from build123d import *

# Parameters (mm, degrees)
SKETCH1_W                          = 155
SKETCH1_H                          = 209.16
BACKPLATE_DEPTH                    = 1.016
IO_SHIELD_CUTOUT_REACH             = 262.334
SKETCH2_W                          = 44.45
SKETCH2_H                          = 158.75
FILLET1_R                          = 0.99
EXPANSION_CARD_CUTOUT_REACH        = 262.334
SKETCH5_W                          = 15
SKETCH5_H                          = 104
SKETCH5_W_2                        = 60.69
SKETCH5_H_2                        = 16
CONVERT_SOLID2_START               = -0.1524
CONVERT_SOLID2_OUTLINE_W           = 155
CONVERT_SOLID2_OUTLINE_H           = 209.16
CONVERT_SOLID2_OUTLINE_W_2         = 15
CONVERT_SOLID2_OUTLINE_H_2         = 104
CONVERT_SOLID2_OUTLINE_W_3         = 60.69
CONVERT_SOLID2_OUTLINE_H_3         = 16
CONVERT_SOLID2_DEPTH               = 0.1524
FILLET2_R                          = 3.048
EXPANSION_CARD_TABS_REACH          = 262.335
SKETCH33_W                         = 15
SKETCH33_H                         = 2
LPATTERN1_COUNT                    = 3
LPATTERN1_PITCH                    = 20.23
M3_CLEARANCE_HOLE_FRAME_MOUNTING_D = 3.4
PANEL_MOUNT_CABLE_CUTOUT_REACH     = 262.335
SKETCH42_W                         = 30.5
SKETCH42_H                         = 22
FILLET3_R                          = 1.5
TAP_DRILL_FOR_M3X0_5_TAP1_D        = 2.5
FILLET4_R                          = 2
FILLET5_R                          = 1
SPINE_MOUNTING_HOLES_D             = 3.2
SPINE_MOUNTING_HOLES_DEPTH         = 5
SPINE_MOUNTING_HOLES_TIP           = 0.96137699


# Read off the part's stored shape, not the designer's step: Convert-Solid2
with BuildPart() as part:
    # Sketch1 → backplate (new body)
    with BuildSketch(Plane.XY):
        with Locations((77.5, 104.58)):
            Rectangle(SKETCH1_W, SKETCH1_H)
    extrude(amount=BACKPLATE_DEPTH)

    # Sketch2 → io_shield_cutout (cut, up to next)
    with BuildSketch(Plane.XY.offset(1.016), mode=Mode.PRIVATE) as io_shield_cutout_sk1:
        with Locations((58.945, 81.955)):
            Rectangle(SKETCH2_W, SKETCH2_H)
    io_shield_cutout_tool1 = extrude(io_shield_cutout_sk1.sketch, amount=-IO_SHIELD_CUTOUT_REACH, mode=Mode.PRIVATE) & part.part
    add(io_shield_cutout_tool1.solids().sort_by_distance((58.945, 81.955, 1.016))[0], mode=Mode.SUBTRACT)

    # Fillet1
    fillet1_edges = [part.edges().sort_by_distance(p)[0] for p in [
        (36.72, 2.58, 0.508),
        (36.72, 161.33, 0.508),
        (81.17, 161.33, 0.508),
        (81.17, 2.58, 0.508),
    ]]
    fillet(fillet1_edges, radius=FILLET1_R)

    # Sketch5 → expansion-card-cutout (cut, up to next)
    with BuildSketch(Plane.XY.offset(1.016), mode=Mode.PRIVATE) as expansion_card_cutout_sk1:
        with Locations((103.88, 89)):
            Rectangle(SKETCH5_W, SKETCH5_H)
    expansion_card_cutout_tool1 = extrude(expansion_card_cutout_sk1.sketch, amount=-EXPANSION_CARD_CUTOUT_REACH, mode=Mode.PRIVATE) & part.part
    # Sketch5 → expansion-card-cutout (cut, up to next)
    with BuildSketch(Plane.XY.offset(1.016), mode=Mode.PRIVATE) as expansion_card_cutout_sk2:
        with Locations((121.835, 153)):
            Rectangle(SKETCH5_W_2, SKETCH5_H_2)
    expansion_card_cutout_tool2 = extrude(expansion_card_cutout_sk2.sketch, amount=-EXPANSION_CARD_CUTOUT_REACH, mode=Mode.PRIVATE) & part.part
    # Sketch5 → expansion-card-cutout (cut, up to next)
    with BuildSketch(Plane.XY.offset(1.016), mode=Mode.PRIVATE) as expansion_card_cutout_sk3:
        with Locations((124.2, 89)):
            Rectangle(SKETCH5_W, SKETCH5_H)
    expansion_card_cutout_tool3 = extrude(expansion_card_cutout_sk3.sketch, amount=-EXPANSION_CARD_CUTOUT_REACH, mode=Mode.PRIVATE) & part.part
    # Sketch5 → expansion-card-cutout (cut, up to next)
    with BuildSketch(Plane.XY.offset(1.016), mode=Mode.PRIVATE) as expansion_card_cutout_sk4:
        with Locations((144.52, 89)):
            Rectangle(SKETCH5_W, SKETCH5_H)
    expansion_card_cutout_tool4 = extrude(expansion_card_cutout_sk4.sketch, amount=-EXPANSION_CARD_CUTOUT_REACH, mode=Mode.PRIVATE) & part.part
    add(expansion_card_cutout_tool1.solids().sort_by_distance((103.88, 89, 1.016))[0], mode=Mode.SUBTRACT)
    add(expansion_card_cutout_tool2.solids().sort_by_distance((121.835, 153, 1.016))[0], mode=Mode.SUBTRACT)
    add(expansion_card_cutout_tool3.solids().sort_by_distance((124.2, 89, 1.016))[0], mode=Mode.SUBTRACT)
    add(expansion_card_cutout_tool4.solids().sort_by_distance((144.52, 89, 1.016))[0], mode=Mode.SUBTRACT)

    # Convert-Solid2 outline → Convert-Solid2 (add)
    with BuildSketch(Plane.XY.offset(CONVERT_SOLID2_START)):
        with Locations((77.5, 104.58)):
            Rectangle(CONVERT_SOLID2_OUTLINE_W, CONVERT_SOLID2_OUTLINE_H)
        with BuildLine():
            ThreePointArc((37.71, 2.58), (37.009964287, 2.869964287), (36.72, 3.57))
            Line((36.72, 3.57), (36.72, 160.34))
            ThreePointArc((36.72, 160.34), (37.009964287, 161.040035713), (37.71, 161.33))
            Line((37.71, 161.33), (80.18, 161.33))
            ThreePointArc((80.18, 161.33), (80.880035713, 161.040035713), (81.17, 160.34))
            Line((81.17, 160.34), (81.17, 3.57))
            ThreePointArc((81.17, 3.57), (80.880035713, 2.869964287), (80.18, 2.58))
            Line((80.18, 2.58), (37.71, 2.58))
        make_face(mode=Mode.SUBTRACT)
        with Locations((103.88, 89)):
            Rectangle(CONVERT_SOLID2_OUTLINE_W_2, CONVERT_SOLID2_OUTLINE_H_2, mode=Mode.SUBTRACT)
        with Locations((124.2, 89)):
            Rectangle(CONVERT_SOLID2_OUTLINE_W_2, CONVERT_SOLID2_OUTLINE_H_2, mode=Mode.SUBTRACT)
        with Locations((144.52, 89)):
            Rectangle(CONVERT_SOLID2_OUTLINE_W_2, CONVERT_SOLID2_OUTLINE_H_2, mode=Mode.SUBTRACT)
        with Locations((121.835, 153)):
            Rectangle(CONVERT_SOLID2_OUTLINE_W_3, CONVERT_SOLID2_OUTLINE_H_3, mode=Mode.SUBTRACT)
    extrude(amount=CONVERT_SOLID2_DEPTH)

    # Fillet2
    fillet2_edges = [part.edges().sort_by_distance(p)[0] for p in [
        (0, 0, 0.4318),
        (0, 209.16, 0.4318),
        (155, 209.16, 0.4318),
        (155, 0, 0.4318),
    ]]
    fillet(fillet2_edges, radius=FILLET2_R)

    # Sketch33 → expansion-card-tabs (cut, up to next)
    with BuildSketch(Plane.XY.offset(1.016), mode=Mode.PRIVATE) as expansion_card_tabs_sk1:
        with Locations((103.88, 32)):
            Rectangle(SKETCH33_W, SKETCH33_H)
    expansion_card_tabs_tool1 = extrude(expansion_card_tabs_sk1.sketch, amount=-EXPANSION_CARD_TABS_REACH, mode=Mode.PRIVATE) & part.part
    # Sketch33 → expansion-card-tabs (cut, up to next)
    with BuildSketch(Plane.XY.offset(1.016), mode=Mode.PRIVATE) as expansion_card_tabs_sk2:
        with Locations((103.88, 28.5)):
            Rectangle(SKETCH33_W, SKETCH33_H)
    expansion_card_tabs_tool2 = extrude(expansion_card_tabs_sk2.sketch, amount=-EXPANSION_CARD_TABS_REACH, mode=Mode.PRIVATE) & part.part
    expansion_card_tabs_1 = expansion_card_tabs_tool1.solids().sort_by_distance((103.88, 32, 1.016))[0]
    add(expansion_card_tabs_1, mode=Mode.SUBTRACT)
    expansion_card_tabs_2 = expansion_card_tabs_tool2.solids().sort_by_distance((103.88, 28.5, 1.016))[0]
    add(expansion_card_tabs_2, mode=Mode.SUBTRACT)
    expansion_card_tabs = expansion_card_tabs_1 + expansion_card_tabs_2  # expansion-card-tabs as one shape, for the pattern or mirror that repeats it

    # LPattern1: expansion-card-tabs ×3
    with Locations(*[(i * LPATTERN1_PITCH, 0, 0) for i in range(1, LPATTERN1_COUNT)]):
        add(expansion_card_tabs, mode=Mode.SUBTRACT)

    # M3 Clearance Hole frame mounting (through all)
    with Locations(Plane(origin=(0, 0, -0.1524), x_dir=(-1, 0, 0), z_dir=(0, 0, -1))):
        with Locations((-12.6, 7.025), (-141, 176.135), (-141, 7.025), (-12.6, 176.135)):
            Hole(M3_CLEARANCE_HOLE_FRAME_MOUNTING_D / 2)

    # Sketch42 → panel-mount-cable-cutout (cut, up to next)
    with BuildSketch(Plane.XY.offset(1.016), mode=Mode.PRIVATE) as panel_mount_cable_cutout_sk1:
        with Locations((120.9, 13.54)):
            Rectangle(SKETCH42_W, SKETCH42_H)
    panel_mount_cable_cutout_tool1 = extrude(panel_mount_cable_cutout_sk1.sketch, amount=-PANEL_MOUNT_CABLE_CUTOUT_REACH, mode=Mode.PRIVATE) & part.part
    add(panel_mount_cable_cutout_tool1.solids().sort_by_distance((120.9, 13.54, 1.016))[0], mode=Mode.SUBTRACT)

    # Fillet3
    fillet3_edges = [part.edges().sort_by_distance(p)[0] for p in [
        (105.65, 2.54, 0.4318),
        (105.65, 24.54, 0.4318),
        (136.15, 24.54, 0.4318),
        (136.15, 2.54, 0.4318),
    ]]
    fillet(fillet3_edges, radius=FILLET3_R)

    # Tap Drill for M3x0.5 Tap1 (through all)
    with Locations(Plane(origin=(100.8, 13.54, 1.016), x_dir=(1, 0, 0), z_dir=(0, 0, 1))):
        with Locations((0, 0), (40.2, 0)):
            Hole(TAP_DRILL_FOR_M3X0_5_TAP1_D / 2)

    # Fillet4
    fillet4_edges = [part.edges().sort_by_distance(p)[0] for p in [
        (91.49, 145, 0.4318),
        (152.18, 145, 0.4318),
        (152.18, 161, 0.4318),
        (91.49, 161, 0.4318),
        (137.02, 37, 0.4318),
        (152.02, 37, 0.4318),
        (152.02, 141, 0.4318),
        (137.02, 141, 0.4318),
        (116.7, 37, 0.4318),
        (131.7, 37, 0.4318),
        (131.7, 141, 0.4318),
        (116.7, 141, 0.4318),
        (96.38, 37, 0.4318),
        (111.38, 37, 0.4318),
        (111.38, 141, 0.4318),
        (96.38, 141, 0.4318),
    ]]
    fillet(fillet4_edges, radius=FILLET4_R)

    # Fillet5
    fillet5_edges = [part.edges().sort_by_distance(p)[0] for p in [
        (116.61, 33, 0.4318),
        (116.61, 31, 0.4318),
        (116.61, 27.5, 0.4318),
        (136.84, 33, 0.4318),
        (136.84, 31, 0.4318),
        (136.84, 27.5, 0.4318),
        (116.61, 29.5, 0.4318),
        (136.84, 29.5, 0.4318),
        (131.61, 27.5, 0.4318),
        (131.61, 29.5, 0.4318),
        (131.61, 33, 0.4318),
        (151.84, 33, 0.4318),
        (151.84, 27.5, 0.4318),
        (151.84, 29.5, 0.4318),
        (151.84, 31, 0.4318),
        (131.61, 31, 0.4318),
        (111.38, 31, 0.4318),
        (111.38, 27.5, 0.4318),
        (111.38, 29.5, 0.4318),
        (96.38, 29.5, 0.4318),
        (96.38, 27.5, 0.4318),
        (96.38, 31, 0.4318),
        (96.38, 33, 0.4318),
        (111.38, 33, 0.4318),
    ]]
    fillet(fillet5_edges, radius=FILLET5_R - 0.0001)  # a hair under: the kernel refuses the full size

    # spine-mounting-holes
    with Locations(Plane.XY.offset(1.016)):
        with Locations((83.71, 176.135), (85.42, 7.025)):
            Hole(SPINE_MOUNTING_HOLES_D / 2, depth=SPINE_MOUNTING_HOLES_DEPTH)
            with Locations((0, 0, -(SPINE_MOUNTING_HOLES_DEPTH + SPINE_MOUNTING_HOLES_TIP / 2))):  # 118° drill point
                Cone(0, SPINE_MOUNTING_HOLES_D / 2, SPINE_MOUNTING_HOLES_TIP, mode=Mode.SUBTRACT)


solid = part.part
Input: part model. Units: mm. Frame: model coordinates. Round coordinates to 2 decimals unless told otherwise and drop trailing zeros. Write each loop counter-clockwise with the first axis right and the second up, starting at its lowest first coordinate (ties: lowest second). Pieces come first, ordered by that corner, then holes.
1) Cut plane A-A (x = 65.5). Return the cut outline in (y, z).
2) Cut plane C-C (z = 0.25). Count the separate pieces of the cut face and the enclosed holes in it, then the cut area to 3 significant figures.
3) Cut plane B-B (y = 109.5). Return the cut outline in (x, z).
4) Contact query for a flat-ended pin moving along its axis: P1, Ø2, axis at x = 100.8, y = 13.54, coming from the +Z side. Output: stop coordinate, or through.
5) Ray query, L1, parallel to X at y = 54.5, z = 0.3; L2, parallel to X at y = 19, z = 0.8; L3, parallel to X at y = 159, z = 0.5. Return the intervals inside material, ascending.
Geometry says:
1. outline: (0, -0.15) - (2.58, -0.15) - (2.58, 1.02) - (0, 1.02) - close; (161.33, -0.15) - (209.16, -0.15) - (209.16, 1.02) - (161.33, 1.02) - close
2. separate pieces: 1
2. enclosed holes: 20
2. area: 18,800 mm2
3. outline: (0, -0.15) - (36.72, -0.15) - (36.72, 1.02) - (0, 1.02) - close; (81.17, -0.15) - (96.38, -0.15) - (96.38, 1.02) - (81.17, 1.02) - close; (111.38, -0.15) - (116.7, -0.15) - (116.7, 1.02) - (111.38, 1.02) - close; (131.7, -0.15) - (137.02, -0.15) - (137.02, 1.02) - (131.7, 1.02) - close; (152.02, -0.15) - (155, -0.15) - (155, 1.02) - (152.02, 1.02) - close
4. P1: passes through
5. L1: x = 0 to 36.72, 81.17 to 96.38, 111.38 to 116.7, 131.7 to 137.02, 152.02 to 155
5. L2: x = 0 to 36.72, 81.17 to 105.65, 136.15 to 155
5. L3: x = 0 to 36.72, 81.17 to 91.49, 152.18 to 155
